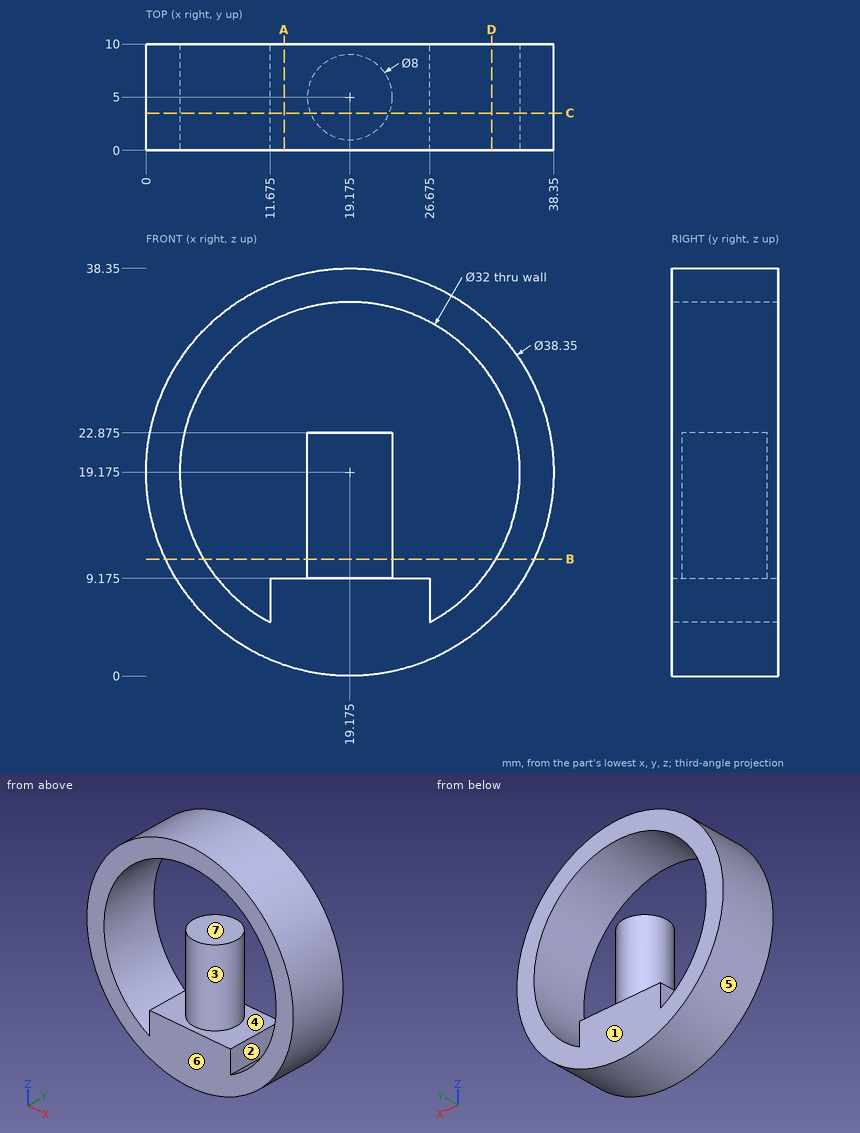
Source: three-view drawing plus pictorial views. Frame: mm from the lowest corner of the part. A direction names the side the tool comes from. Round coordinates to 2 decimals unless told otherwise and drop trailing zeros. Order: outer loops, then holes, each group sorted by start corner. A loop starts at its lowest first (then second) coordinate and runs counter-clockwise, first axis right, second up. Notation, with made-up numbers: (23.5, -35.5) - (61.5, -35.5) arc R37 ccw to (61.5, 3.5) - close; hole circle Ø11 at (7, -6). An arc over 180 degrees is marked (long way). Use a Markdown table: item, result.
1. Access query for the marked faces 1, 2 and 3. Directions: +Z, -Z, +X, -X, +Y, -Y. A direction counts if a zero-diameter tool reaches every point of the face in a straight line with its end or side. Return the directions, or none.
Evaluation:
| item | result |
|---|---|
| face 1 | +Z, -Z, +X, -X, +Y |
| face 2 | +Y, -Y |
| face 3 | none |
2. Section C-C on y = 3.5. Return the cut outline in (x, z) (3 decimals).
Evaluation:
| item | result |
|---|---|
| outline | circle Ø38.35 at (19.175, 19.175); hole (11.675, 5.042) - (11.675, 9.175) - (15.467, 9.175) - (15.467, 22.875) - (22.883, 22.875) - (22.883, 9.175) - (26.675, 9.175) - (26.675, 5.042) arc R16 ccw (long way) to start |
3. Section B-B on z = 11. Return the cut outline in (x, y) (3 decimals), then the cut area to 3 significant figures.
Evaluation:
| item | result |
|---|---|
| outline | (1.83, 0) - (5.421, 0) - (5.421, 10) - (1.83, 10) - close; circle Ø8 at (19.175, 5); (32.929, 0) - (36.52, 0) - (36.52, 10) - (32.929, 10) - close |
| area | 122 mm^2 |
4. Mould query, pull axis Z, two halves, no side actions, for the marked faces 4, 5, 6 and 7. Classes: +Z half, -Z half, draft (parallel to the pull), parting line (faces both ways), or undercut.
Evaluation:
| item | result |
|---|---|
| face 4 | undercut |
| face 5 | parting line |
| face 6 | draft |
| face 7 | undercut |
5. Section A-A on x = 13. Return the cut outline in (y, z) (3 decimals).
Evaluation:
| item | result |
|---|---|
| outline | (0, 1.021) - (10, 1.021) - (10, 9.175) - (0, 9.175) - close; (0, 33.935) - (10, 33.935) - (10, 37.329) - (0, 37.329) - close |
6. Material intervals for probe 1 along X at (y, z) = (5.75, 20); probe 2 along X at (y, z) = (7.75, 8.5) (3 decimals); probe 3 along Y at (x, z) = (19, 19), sorted ascending.
Evaluation:
| item | result |
|---|---|
| probe 1 | 0.02 to 3.2, 15.25 to 23.1, 35.15 to 38.33 |
| probe 2 | 3.246 to 7.257, 11.675 to 26.675, 31.093 to 35.104 |
| probe 3 | 1 to 9 |
7. Section D-D on x = 32.5. Return the cut outline in (y, z).
Evaluation:
| item | result |
|---|---|
| outline | (0, 5.39) - (10, 5.39) - (10, 10.32) - (0, 10.32) - close; (0, 28.03) - (10, 28.03) - (10, 32.96) - (0, 32.96) - close |
8. First-contact query: pin 1 (1.2 mm diameter, centred on y = 4.5, z = 7, fed in from -X); pin 2 (4.5 mm diameter, centred on y = 4.5, z = 8, fed in from +X); pin 3 (5 mm diameter, centred on y = 2, z = 15, fed in from +X). Flat tips, straight axial feed; report the tip coordinate or a pass-through.
Evaluation:
| item | result |
|---|---|
| pin 1 | x = 3.89 |
| pin 2 | x = 36.15 |
| pin 3 | x = 38.28 |
